Source: three-view drawing plus pictorial views. Frame: mm from the lowest corner of the part. Give positions to 0.01 mm unless a question says otherwise; leave off trailing zeros. Loops run counter-clockwise (first coordinate to the right, second up) from the corner with the lowest first, then second, coordinate; pieces in that order, holes last. Notation, with made-up numbers: (21, 2) - (47, 2) arc R19 cw to (47, 30) - close; hole circle Ø4 at (86.25, 12.5). An arc over 180 degrees is marked (long way). Answer in a Markdown table with one row per item.
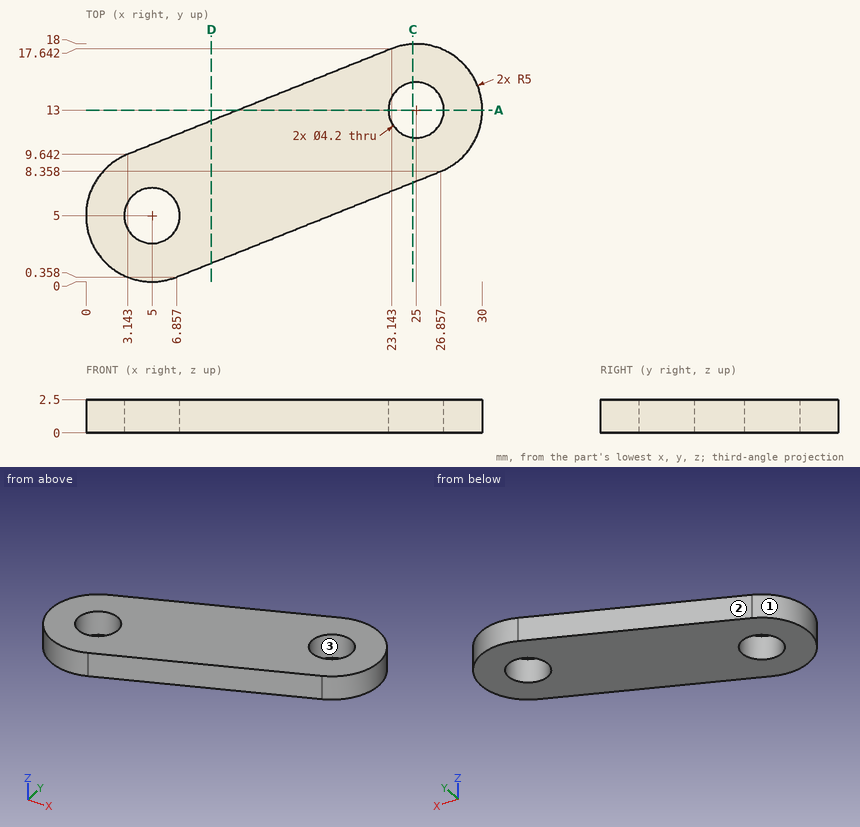
Q1. Cut plane C-C (x = 24.75). Output: boundary loops of the cut face in (y, z) (1 decimal).
Check values:
| item | result |
|---|---|
| outline | (7.5, 0) - (10.9, 0) - (10.9, 2.5) - (7.5, 2.5) - close; (15.1, 0) - (18, 0) - (18, 2.5) - (15.1, 2.5) - close |
Q2. Draft query along Y for the marked faces 1, 2 and 3. Return one class per face: pulls with the +Y half, pulls with the -Y half, needs draft (parallel to the pull), parting line crosses it, or undercut.
Check values:
| item | result |
|---|---|
| face 1 | parting line crosses it |
| face 2 | pulls with the +Y half |
| face 3 | undercut |
Q3. Cut plane A-A (y = 13). Output: boundary loops of the cut face in (x, z).
Check values:
| item | result |
|---|---|
| outline | (11.54, 0) - (22.9, 0) - (22.9, 2.5) - (11.54, 2.5) - close; (27.1, 0) - (30, 0) - (30, 2.5) - (27.1, 2.5) - close |
Q4. Material intervals for line 1 along Y through (x, z) = (25.75, 1.3) (1 decimal); line 2 along Y through (x, z) = (25.25, 2) (1 decimal); line 3 along X through (y, z) = (13, 1.9) (1 decimal), sorted ascending.
Check values:
| item | result |
|---|---|
| line 1 | 7.9 to 11, 15 to 17.9 |
| line 2 | 7.7 to 10.9, 15.1 to 18 |
| line 3 | 11.5 to 22.9, 27.1 to 30 |
Q5. Cut plane D-D (x = 9.5). Output: boundary loops of the cut face in (y, z) (1 decimal).
Check values:
| item | result |
|---|---|
| outline | (1.4, 0) - (12.2, 0) - (12.2, 2.5) - (1.4, 2.5) - close |
